Part model, mm, in its own coordinate system. Face numbers are marked on the shaded views. A direction names the side the tool comes from. Give positions to 0.01 mm unless a question says otherwise; leave off trailing zeros. Write each loop counter-clockwise with the first axis right and the second up, starting at its lowest first coordinate (ties: lowest second). Pieces come first, ordered by that corner, then holes. Notation, with made-up numbers: M 27.25,70 L 50.25,70 A15 ccw 50.25,74 Z; hole C 69,34 d2. An arc over 180 degrees is marked long. Use CSV: the item, a comma, the result in double quotes. Start each with the question number.
1. Drop flat-ended pins along their axis: pin 1 Ø11 at (x, y) = (44, -1) entering from +Z; pin 2 Ø3.5 at (x, z) = (49, 14) entering from -Y; pin 3 Ø6 at (x, z) = (75, -8.5) entering from +Y (3 decimals). Give the stop position or say it passes through.
2. Drill centre lines: line 1 along X through (y, z) = (10.5, -16.5); line 2 along X through (y, z) = (-11, -7.5); line 3 along Z through (x, y) = (84.5, -10). Where is each one in solid material? Low to high. Write a range as from..to.
3. 3-axis set-ups, long thin cutter, end or side, ignore diameter. For the marked faces 1, 2 and 3: which of +Z, -Z, +X, -X, +Y, -Y reach the whole face in a straight line?
4. Band-saw the part on A-A, the plane x = 114.5. List the corners of the cut face in (y, z).
from build123d import *

# Parameters (mm, degrees)
TAGLIO_ESTRUSIONE1_DEPTH = 5
SMUSSO1_SIZE             = 1
SMUSSO2_SIZE             = 1
SMUSSO3_SIZE             = 1
RACCORDO3_R              = 1


with BuildPart() as part:
    # Schizzo1 → Rivoluzione1 (revolve)
    with BuildSketch(Plane.XY, mode=Mode.PRIVATE) as rivoluzione1_sk:
        Polygon((0, 0), (0, 12.5), (3.6, 12.5), (3.6, 11.95), (5, 11.95), (5.317542648, 12.5), (23, 12.5), (23, 16), (29.8, 16), (29.8, 15.15), (31.5, 15.15), (31.990747729, 16), (111.5, 16), (111.5, 20), (116, 20), (116, 16), (120, 16), (120, 12.5), (134.682457352, 12.5), (135, 11.95), (136.4, 11.95), (136.4, 12.5), (140, 12.5), (140, 0), align=None)
    revolve(rivoluzione1_sk.sketch.rotate(Axis((0, 0, 0), (1, 0, 0)), 90), axis=Axis((0, 0, 0), (1, 0, 0)))

    # Schizzo2 → Taglio-Estrusione1 (cut)
    with BuildSketch(Plane.XY.offset(16)):
        with BuildLine():
            Line((40.5, 5), (60.5, 5))
            ThreePointArc((60.5, 5), (65.5, 0), (60.5, -5))
            Line((60.5, -5), (40.5, -5))
            ThreePointArc((40.5, -5), (35.5, 0), (40.5, 5))
        make_face()
        with BuildLine():
            Line((85.5, 5), (103.5, 5))
            ThreePointArc((103.5, 5), (108.5, 0), (103.5, -5))
            Line((103.5, -5), (85.5, -5))
            ThreePointArc((85.5, -5), (80.5, 0), (85.5, 5))
        make_face()
    extrude(amount=-TAGLIO_ESTRUSIONE1_DEPTH, mode=Mode.SUBTRACT)

    # Smusso1
    smusso1_edges = [part.edges().sort_by_distance(p)[0] for p in [
        (0, 0, -12.5),
    ]]
    chamfer(smusso1_edges, length=SMUSSO1_SIZE)

    # Smusso2
    smusso2_edges = [part.edges().sort_by_distance(p)[0] for p in [
        (140, 0, -12.5),
    ]]
    chamfer(smusso2_edges, length=SMUSSO2_SIZE)

    # Smusso3
    smusso3_edges = [part.edges().sort_by_distance(p)[0] for p in [
        (120, 0, -16),
        (23, 0, -16),
    ]]
    chamfer(smusso3_edges, length=SMUSSO3_SIZE)

    # Raccordo3
    raccordo3_edges = [part.edges().sort_by_distance(p)[0] for p in [
        (116, 0, -16),
        (111.5, 0, -16),
    ]]
    fillet(raccordo3_edges, radius=RACCORDO3_R)


solid = part.part
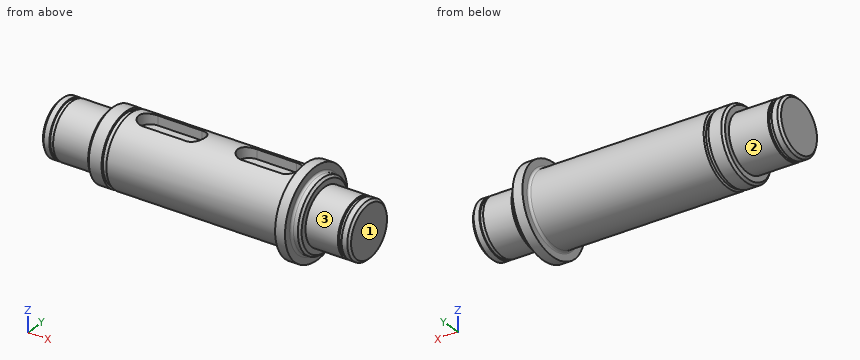
Output:
1,pin 1,"stops at z = 15.2"
1,pin 2,"stops at y = -10.29"
1,pin 3,"stops at y = 15.025"
2,line 1,"x = 111.5..116"
2,line 2,"x = 23..120"
2,line 3,"z = -12.49..12.49"
3,face 1,"+Z, -Z, +X, +Y, -Y"
3,face 2,"-X"
3,face 3,"+X"
4,outline,"C 0,0 d40"
